from build123d import *

# Parameters (mm, degrees)
BOSS_EXTRUDE1_DEPTH        = 80
F_5_5_5_5_DIAMETER_HOLE1_D = 5.5
F_8_5_8_5_DIAMETER_HOLE1_D = 8.5


with BuildPart() as part:
    # Sketch1 → Boss-Extrude1 (new body)
    with BuildSketch(Plane(origin=(0, 0, 0), x_dir=(1, 0, 0), z_dir=(0, 1, 0))):
        Polygon((0, 0), (40, 0), (40, -4), (4, -4), (4, -40), (0, -40), align=None)
    extrude(amount=BOSS_EXTRUDE1_DEPTH)

    # Ø5.5 (5.5) Diameter Hole1 (through all)
    with Locations(Plane.XY.offset(4)):
        with Locations((32.5, 70), (15, 70), (15, 50), (32.5, 50), (32.5, 30), (15, 30), (15, 10), (32.5, 10)):
            Hole(F_5_5_5_5_DIAMETER_HOLE1_D / 2)

    # Ø8.5 (8.5) Diameter Hole1 (through all)
    with Locations(Plane(origin=(4, 0, 0), x_dir=(0, 0, -1), z_dir=(1, 0, 0))):
        with Locations((-22.5, 70), (-22.5, 10)):
            Hole(F_8_5_8_5_DIAMETER_HOLE1_D / 2)


solid = part.part
The listing builds one solid part. Answer for the finished solid, in the listing's coordinates (mm). A direction names the side the tool comes from. Round coordinates to 2 decimals unless told otherwise and drop trailing zeros. Write each loop counter-clockwise with the first axis right and the second up, starting at its lowest first coordinate (ties: lowest second). Pieces come first, ordered by that corner, then holes. Notation, with made-up numbers: (56, -32.5) - (84, -32.5) arc R23 ccw to (84, -15.5) - close; hole circle Ø7 at (42.5, 41.25). An arc over 180 degrees is marked (long way). Use one line per item in the form item = value. Start each with the question number.
Item 1: Flat-ended cylindrical pins translate along their axes: pin 1 Ø4 at (x, y) = (28.5, 26) entering from -Z; pin 2 Ø11 at (x, y) = (16, 34) entering from +Z; pin 3 Ø2 at (y, z) = (36, 9.5) entering from +X. Find the tip coordinate at first contact, or state that the pin passes through.
Item 2: A cutting plane is placed at D-D (y = 10). Write down the section's boundary in (x, z).
Item 3: Determine the mould class of faces 1 (the flat face through (20, 39, 0)), 2 (the flat face through (2, 39, 40)), 3 (the cylindrical face through (15.358, 32.727, 1.972)), 4 (the cylindrical face through (1.97, 5.85, 21.58)) for opening direction Z: +Z half, -Z half, draft (parallel to the pull), parting line (faces both ways), or undercut.
Item 4: A cutting plane is placed at B-B (z = 22.5). Write down the section's boundary in (x, y).
Item 5: Find the intervals of material crossed by line 1 (Y direction, x = 32, z = 2); line 2 (Z direction, x = 32.5, y = 17), in increasing order. Write a range as [from, to].
Item 6: A tool of negligible diameter and unlimited length cuts with its end or side. For faces 5 (the flat face through (40, 39, 2)), 6 (the flat face through (4, 39, 22)), from which of +Z, -Z, +X, -X, +Y, -Y can it reach the whole face along a straight path? Write none if from no direction.
Item 7: A cutting plane is placed at C-C (y = 50). Write down the section's boundary in (x, z).
Item 8: A cutting plane is placed at A-A (x = 32.5). Write down the section's boundary in (y, z), plus the area to 3 significant figures.
The answers:
q1.pin_1 = 0
q1.pin_2 = 4
q1.pin_3 = 4
q2.outline = (0, 0) - (12.25, 0) - (12.25, 4) - (4, 4) - (4, 18.25) - (0, 18.25) - close; (0, 26.75) - (4, 26.75) - (4, 40) - (0, 40) - close; (17.75, 0) - (29.75, 0) - (29.75, 4) - (17.75, 4) - close; (35.25, 0) - (40, 0) - (40, 4) - (35.25, 4) - close
q3.face_1 = -Z half
q3.face_2 = +Z half
q3.face_3 = draft
q3.face_4 = undercut
q4.outline = (0, 0) - (4, 0) - (4, 5.75) - (0, 5.75) - close; (0, 14.25) - (4, 14.25) - (4, 65.75) - (0, 65.75) - close; (0, 74.25) - (4, 74.25) - (4, 80) - (0, 80) - close
q5.line_1 = [0, 7.3], [12.7, 27.3], [32.7, 47.3], [52.7, 67.3], [72.7, 80]
q5.line_2 = [0, 4]
q6.face_5 = +Z, -Z, +X, +Y, -Y
q6.face_6 = +Z, +X, +Y, -Y
q7.outline = (0, 0) - (12.25, 0) - (12.25, 4) - (4, 4) - (4, 40) - (0, 40) - close; (17.75, 0) - (29.75, 0) - (29.75, 4) - (17.75, 4) - close; (35.25, 0) - (40, 0) - (40, 4) - (35.25, 4) - close
q8.outline = (0, 0) - (7.25, 0) - (7.25, 4) - (0, 4) - close; (12.75, 0) - (27.25, 0) - (27.25, 4) - (12.75, 4) - close; (32.75, 0) - (47.25, 0) - (47.25, 4) - (32.75, 4) - close; (52.75, 0) - (67.25, 0) - (67.25, 4) - (52.75, 4) - close; (72.75, 0) - (80, 0) - (80, 4) - (72.75, 4) - close
q8.area = 232 mm^2
